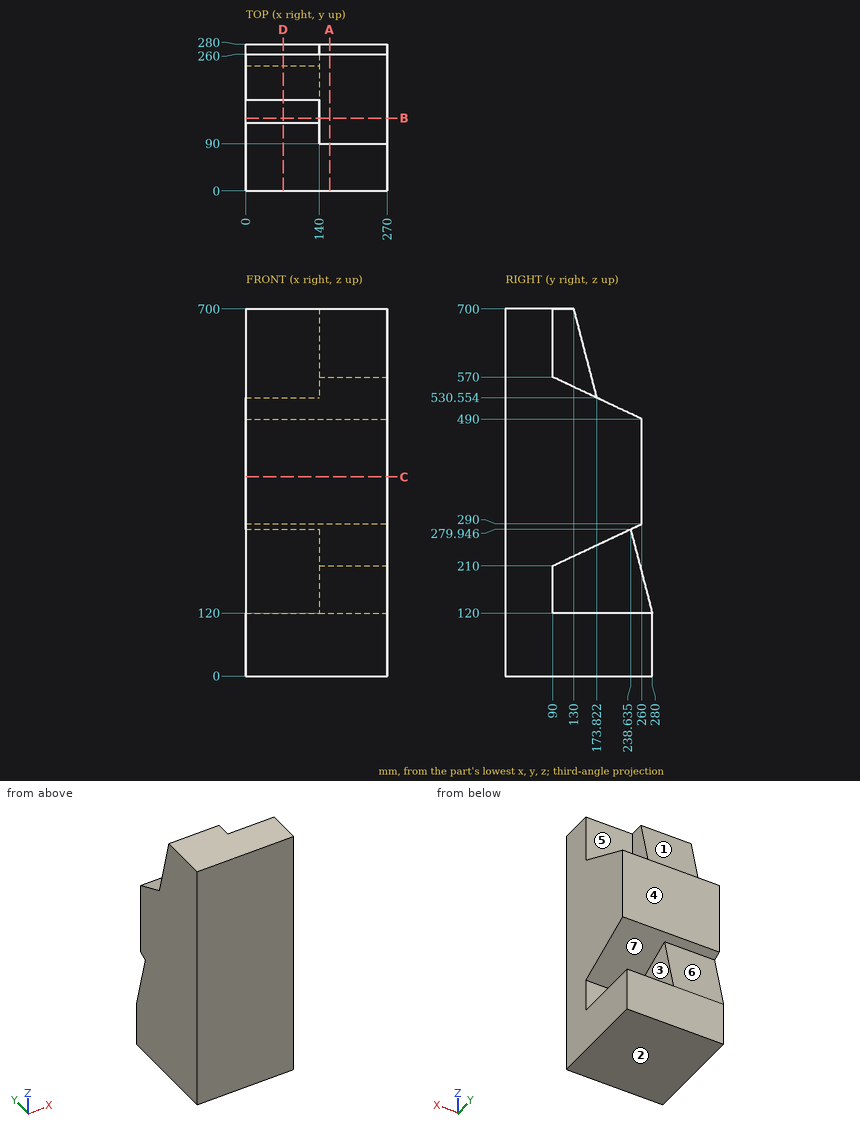
Geometry check sheet. Reference: drawing and pictorial views, mm from the part's lowest x, y, z. A direction names the side the tool comes from. Round coordinates to 2 decimals unless told otherwise and drop trailing zeros. Loops run counter-clockwise (first coordinate to the right, second up) from the corner with the lowest first, then second, coordinate; pieces in that order, holes last. Notation, with made-up numbers: (7.5, -33.75) - (22.5, -33.75) arc R28 cw to (22.5, -5.75) - close; hole circle Ø8 at (-15, -4). An arc over 180 degrees is marked (long way). Write item = value, one per line. Start each with the question number.
Q1. Section check C-C (z = 379.5). Record the boundary of the cut face in (x, y), plus the area to 3 significant figures.
Q2. Depth check by flat-ended pin: P1, Ø1, axis at x = 211, z = 470, coming from the +Y side; P2, Ø25, axis at y = 143, z = 646.5, coming from the +X side. Enter the tip coordinate at first touch or a pass-through.
Q3. Section check B-B (y = 138.5). Record the boundary of the cut face in (x, z).
Q4. Section check A-A (x = 160). Record the boundary of the cut face in (y, z).
Q5. Thickness scan on L1, parallel to Y at x = 144.5, z = 643.5; L2, parallel to X at y = 164.5, z = 144.5; L3, parallel to Y at x = 221.5, z = 427. Record the ranges inside material, lowest first.
Q6. Access from +Z, -Z, +X, -X, +Y, -Y to the whole of each face (thin tool, end or side, straight path). Record for the marked faces 4, 5, 6 and 7.
Q7. Section check D-D (x = 71). Record the boundary of the cut face in (y, z) (1 decimal).
Q8. Release check for a two-part mould opening along Z. For the marked faces 1, 2 and 3 record: pulls with the +Z half, pulls with the -Z half, needs draft (parallel to the pull), parting line crosses it, or undercut.
Derived:
q1.outline = (0, 0) - (270, 0) - (270, 260) - (0, 260) - close
q1.area = 70,200 mm^2
q2.P1 = 260
q2.P2 = 140
q3.outline = (0, 0) - (270, 0) - (270, 120) - (140, 120) - (140, 232.82) - (270, 232.82) - (270, 547.18) - (140, 547.18) - (140, 667.13) - (0, 667.13) - close
q4.outline = (0, 0) - (280, 0) - (280, 120) - (90, 120) - (90, 210) - (260, 290) - (260, 490) - (90, 570) - (90, 700) - (0, 700) - close
q5.L1 = 0 to 90
q5.L2 = 0 to 140
q5.L3 = 0 to 260
q6.face_4 = +Z, +X, -X, +Y
q6.face_5 = +Z, +X, +Y
q6.face_6 = +X, -X, +Y
q6.face_7 = +X, +Y
q7.outline = (0, 0) - (280, 0) - (280, 120) - (238.6, 279.9) - (260, 290) - (260, 490) - (173.8, 530.6) - (130, 700) - (0, 700) - close
q8.face_1 = pulls with the +Z half
q8.face_2 = pulls with the -Z half
q8.face_3 = undercut
